Build history of the part. All positions in model axes, mm. A direction names the side the tool comes from. Round coordinates to 2 decimals unless told otherwise and drop trailing zeros. Write each loop counter-clockwise with the first axis right and the second up, starting at its lowest first coordinate (ties: lowest second). Pieces come first, ordered by that corner, then holes. Notation, with made-up numbers: (-28, 64.5) - (-13, 64.5) arc R19 cw to (-13, 86.5) - close; hole circle Ø10 at (-38.5, 56.5). An arc over 180 degrees is marked (long way). Write each question's results on one line, items separated by ' | '.
Autodesk Inventor part; units mm, degrees
ref_plane "Work Plane1" through (-26.25, -7, 0) normal (0, -1, 0) x (1, 0, 0)
ref_plane "YZ Plane" through (0, 0, 0) normal (1, 0, 0) x (0, 1, 0)
ref_plane "XZ Plane" through (0, 0, 0) normal (0, 1, 0) x (-1, 0, 0)
sketch "Sketch2" plane through (0, 0, 0) normal (0, 0, 1) x (1, 0, 0)
  line L0 (-26.25, -7) -> (26.25, -7) construction
  line L1 (26.25, -7) -> (26.25, -3)
  line L2 (23.25, 0) -> (-23.25, 0)
  line L3 (-26.25, -3) -> (-26.25, -7)
  arc A0 (-23.25, 0) -> (-26.25, -3) centre (-23.25, -3) ccw
  arc A1 (26.25, -3) -> (23.25, 0) centre (23.25, -3) ccw
  point P0 (0, 0)
  point P1 (26.25, 0)
  point P2 (-26.25, 0)
  point P3 (0, 0)
  dimension "d11" = 52.5
  dimension "d12" = 7
  dimension "d13" = 3
ref_plane "Work Plane1" through (-26.25, -7, 0) normal (0, -1, 0) x (1, 0, 0)
sketch "Sketch3" plane through (-26.25, -7, 0) normal (0, -1, 0) x (1, 0, 0)
  circle A0 centre (0, 0) radius 2.25
  point P0 (26.25, 0)
  dimension "d14" = 4.5
sweep "Sweep1" add profiles "Sketch3" path "Sketch2"
fillet "Fillet1" radius 0.5 6 edges at (28.5, -7, 0) (28.5, -3, 0) (23.25, 2.25, 0) (-23.25, 2.25, 0) (-28.5, -3, 0) (-28.5, -7, 0)
properties part number "Solder Roll Support 3" material "SAE 1020"
(1) Slice it at C-C, the plane x = 7. Write the cut outline in (y, z), and give its area (3 significant figures).
Worked answers:
outline: circle Ø4.5 at (0, 0) | area: 15.9 mm2
(2) Flat gauge pin, fed straight in: pin 1 Ø5 at (x, y) = (-10, -1.5) entering from +Z. Where does the tip first touch, or does it go through?
Worked answers:
pin 1: stops at z = 2.25
(3) Slice it at A-A, the plane y = -4. Write the cut outline in (x, z), and give its area (3 significant figures).
Worked answers:
outline: circle Ø4.5 at (-26.25, 0); circle Ø4.5 at (26.25, 0) | area: 31.8 mm2
(4) Tool access for faces 1 (the cylindrical face through (-24.104, -4.774, 0.676)), 2 (the flat face through (-26, -7, 0)), 3 (the cylindrical face through (-0.33, 0.29, 2.23)): list every direction of +Z, -Z, +X, -X, +Y, -Y with a clear straight run to the whole face (end or side of a thin tool).
Worked answers:
face 1: -Y | face 2: +Z, -Z, +X, -X, -Y | face 3: none
(5) Slice it at B-B, the plane z = 0. Write the cut outline in (x, y).
Worked answers:
outline: (-28.5, -6.5) arc R0.5 ccw to (-28, -7) - (-24.5, -7) arc R0.5 ccw to (-24, -6.5) - (-24, -3) arc R0.75 cw to (-23.25, -2.25) - (23.25, -2.25) arc R0.75 cw to (24, -3) - (24, -6.5) arc R0.5 ccw to (24.5, -7) - (28, -7) arc R0.5 ccw to (28.5, -6.5) - (28.5, -3) arc R5.25 ccw to (23.25, 2.25) - (-23.25, 2.25) arc R5.25 ccw to (-28.5, -3) - close
(6) Drill centre lines: probe 1 along Y at (x, z) = (0, -0.2); probe 2 along Z at (x, y) = (26, -2); probe 3 along X at (y, z) = (-3.75, -0.9). Where is each one in solid material? Low to high. Write a range as [from, to].
Worked answers:
probe 1: y = [-2.24, 2.24] | probe 2: z = [-2.25, 2.25] | probe 3: x = [-28.31, -24.19], [24.19, 28.31]
